CAD build for the part. Positions are in the model's coordinates, mm. Face numbers are marked on the shaded views. Give positions to 0.01 mm unless a question says otherwise; leave off trailing zeros. Loops run counter-clockwise (first coordinate to the right, second up) from the corner with the lowest first, then second, coordinate; pieces in that order, holes last. Notation, with made-up numbers: (-18, 13) -> (15, 13) arc R24 cw to (15, 26) -> close; hole circle Ø7 at (-16.75, 41.5). An arc over 180 degrees is marked (long way). Use one line per item in the form item = value.
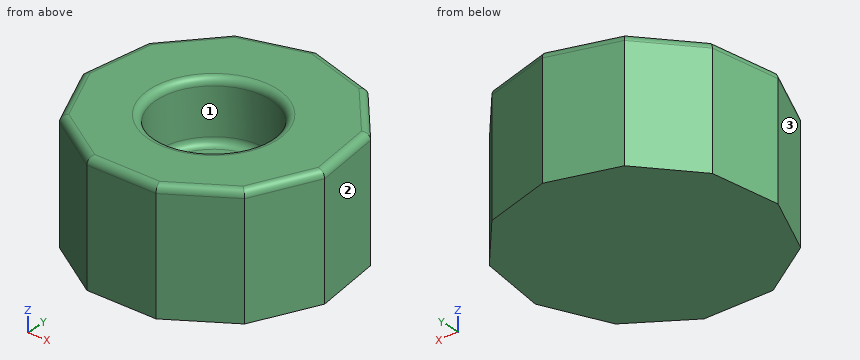
```python
from build123d import *

# Parameters (mm, degrees)
F1_DEPTH = 50.8
F2_R     = 23.7463385983
F3_DEPTH = 25.4
F4_R     = 3


with BuildPart() as f1:
    # F0 (on Top) → F1 (new body)
    with BuildSketch(Plane.XY):
        Polygon((-14.6813246469, -50), (14.6813246469, -50), (39.3827570986, -34.1253532831), (51.5804424368, -7.4161480171), (47.4017017513, 21.6476318444), (28.1732556841, 43.8384415501), (0, 52.1108558113), (-28.1732556841, 43.8384415501), (-47.4017017513, 21.6476318444), (-51.5804424368, -7.4161480171), (-39.3827570986, -34.1253532831), align=None)
    extrude(amount=F1_DEPTH)

    # F2 (on face) → F3 (cut)
    with BuildSketch(Plane.XY.offset(50.8)):
        with Locations((0, -2.0428874996)):
            Circle(F2_R)
    extrude(amount=-F3_DEPTH, mode=Mode.SUBTRACT)

    # F4
    f4_edges = [f1.edges().sort_by_distance(p)[0] for p in [
        (-23.746339, -2.042887, 25.4),
        (-23.746339, -2.042887, 50.8),
        (0, -50, 50.8),
        (-27.032041, -42.062677, 50.8),
        (27.032041, -42.062677, 50.8),
        (-45.4816, -20.770751, 50.8),
        (45.4816, -20.770751, 50.8),
        (-49.491072, 7.115742, 50.8),
        (49.491072, 7.115742, 50.8),
        (-37.787479, 32.743037, 50.8),
        (37.787479, 32.743037, 50.8),
        (-14.086628, 47.974649, 50.8),
        (14.086628, 47.974649, 50.8),
    ]]
    fillet(f4_edges, radius=F4_R)


solid = f1.part
```
1. Cut at A-A, the plane z = 34. Write the cut outline in (x, y), then the cut area to 3 significant figures.
Result sheet:
outline = (-51.58, -7.42) -> (-39.38, -34.13) -> (-14.68, -50) -> (14.68, -50) -> (39.38, -34.13) -> (51.58, -7.42) -> (47.4, 21.65) -> (28.17, 43.84) -> (0, 52.11) -> (-28.17, 43.84) -> (-47.4, 21.65) -> close; hole circle Ø47.49 at (0, -2.04)
area = 6,300 mm^2
2. Drop flat-ended pins along their axis: P1, Ø20.5, axis at x = -8.5, y = 7, coming from the +Z side; P2, Ø10, axis at y = 3, z = 6.5, coming from the +X side; P3, Ø5, axis at x = 33.5, z = 37, coming from the +Y side. Give the stop position or say it passes through.
Result sheet:
P1 = 26.09
P2 = 50.8
P3 = 40.58
3. Drill centre lines: line 1 (Y direction, x = 0, z = 39.75); line 2 (Z direction, x = 3, y = -4); line 3 (X direction, y = -9.5, z = 31). Where is each one in solid material? Low to high.
Result sheet:
line_1 = -50 to -25.79, 21.7 to 52.11
line_2 = 0 to 25.4
line_3 = -50.63 to -22.55, 22.55 to 50.63
4. Mould opens along Y. For the marked faces 1, 2 and 3 say: pulls with the +Y half, pulls with the -Y half, needs draft (parallel to the pull), parting line crosses it, or undercut.
Result sheet:
face_1 = undercut
face_2 = pulls with the +Y half
face_3 = pulls with the -Y half
